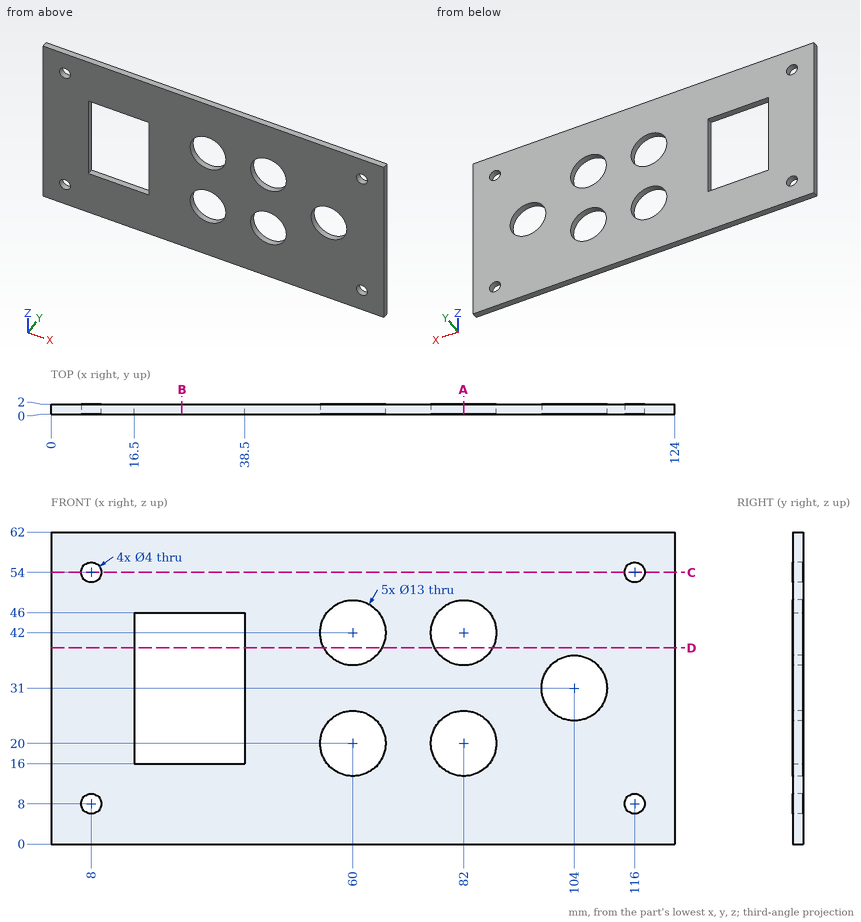
Could you check a few things on this drawing? It's one solid part, dimensions in mm from its lowest x, y, z. Give positions to 0.01 mm unless a question says otherwise; leave off trailing zeros. Loops run counter-clockwise (first coordinate to the right, second up) from the corner with the lowest first, then second, coordinate; pieces in that order, holes last. Notation, with made-up numbers: M 58,-19 L 100,-19 A8 ccw 100,-9 Z; hole C 22.5,47.25 d5. An arc over 180 degrees is marked long. Return JSON: item names as keys, results as strings.
Item 1: Imagine slicing it at D-D on z = 39. List the corners of the cut face in (x, y) for me, then the cut area to 3 significant figures.
A:
{"outline": "M 0,0 L 16.5,0 L 16.5,2 L 0,2 Z; M 38.5,0 L 54.23,0 L 54.23,2 L 38.5,2 Z; M 65.77,0 L 76.23,0 L 76.23,2 L 65.77,2 Z; M 87.77,0 L 124,0 L 124,2 L 87.77,2 Z", "area": "158 mm^2"}
Item 2: Please list where these lines run through material, in increasing order: line 1 (X direction, y = 1.05, z = 8); line 2 (X direction, y = 0.8, z = 20); line 3 (Z direction, x = 82, y = 1.3).
A:
{"line 1": "x = 0 to 6, 10 to 114, 118 to 124", "line 2": "x = 0 to 16.5, 38.5 to 53.5, 66.5 to 75.5, 88.5 to 124", "line 3": "z = 0 to 13.5, 26.5 to 35.5, 48.5 to 62"}
Item 3: Imagine slicing it at A-A on x = 82. List the corners of the cut face in (y, z) for me, then the cut area to 3 significant figures.
A:
{"outline": "M 0,0 L 2,0 L 2,13.5 L 0,13.5 Z; M 0,26.5 L 2,26.5 L 2,35.5 L 0,35.5 Z; M 0,48.5 L 2,48.5 L 2,62 L 0,62 Z", "area": "72.0 mm^2"}
Item 4: Imagine slicing it at B-B on x = 26. List the corners of the cut face in (y, z) for me.
A:
{"outline": "M 0,0 L 2,0 L 2,16 L 0,16 Z; M 0,46 L 2,46 L 2,62 L 0,62 Z"}
Item 5: I'm going to push a flat-ended pin straight in: pin 1 Ø6.5 at (x, z) = (116, 8) entering from +Y. Where does the tip first touch, or does it pass through?
A:
{"pin 1": "stops at y = 2"}
Item 6: Imagine slicing it at C-C on z = 54. List the corners of the cut face in (x, y) for me.
A:
{"outline": "M 0,0 L 6,0 L 6,2 L 0,2 Z; M 10,0 L 114,0 L 114,2 L 10,2 Z; M 118,0 L 124,0 L 124,2 L 118,2 Z"}
